Could you check a few things on this model? Use its own coordinates, in mm. Face numbers are marked on the shaded views. A direction names the side the tool comes from. Round coordinates to 2 decimals unless told otherwise and drop trailing zeros. Write each loop counter-clockwise with the first axis right and the second up, starting at its lowest first coordinate (ties: lowest second). Pieces come first, ordered by that corner, then holes. Notation, with made-up numbers: (42, 2) -> (89, 2) arc R21 ccw to (89, 30) -> close; hole circle Ø9 at (-3.75, -3.75). An arc over 180 degrees is marked (long way). Answer as CSV lines item,"result". Start each with the question number.
Q1. Imagine slicing it at B-B on y = -26.2. Please give me the cut outline in (x, z).
Q2. If we mould it in two halves opening along Y, with no side actions, what happens to the marked faces 1, 2 and 3? For each: pulls with the +Y half, pulls with the -Y half, needs draft (parallel to the pull), parting line crosses it, or undercut.
Q3. Imagine slicing it at A-A on x = 25.3. Please give me the cut outline in (y, z), and give its area (3 significant figures).
Q4. Will these pins go through, and if not, where does the flat tip stop? pin 1 Ø10.5 at (x, y) = (37, 30) entering from -Z; pin 2 Ø9 at (x, y) = (25.3, -26.2) entering from +Z; pin 3 Ø3 at (x, z) = (16.5, 1) entering from +Y; pin 4 Ø12 at (y, z) = (-4, -1) entering from +X.
Q5. Imagine slicing it at C-C on z = 0. Please give me the cut outline in (x, y).
Q6. If I drill on line 1 (X direction, y = -26, z = -6); line 2 (Y direction, x = 25.3, z = -6.6); line 3 (Z direction, x = 10.5, y = 35.5), over which ranges is the centre line in solid material (lowest first)? Write a range as [from, to].
Q7. Imagine slicing it at D-D on y = 0. Please give me the cut outline in (x, z).
Q8. For the marked faces 4, 5 and 6, which set-ups out of +Z, -Z, +X, -X, +Y, -Y let a thin tool reach every point of the face, with its end or its side?
from build123d import *

# Parameters (mm, degrees)
F0_R     = 50
F1_DEPTH = 5
F3_DEPTH = 50
F4_R     = 5
F5_DEPTH = 4


with BuildPart() as f1:
    # F0 (on Right) → F1 (new body)
    with BuildSketch(Plane.YZ):
        Circle(F0_R)
    extrude(amount=-F1_DEPTH)

    # F2 (on Right) → F3 (join)
    with BuildSketch(Plane.YZ):
        Polygon((-41.5, 9), (-41.5, -9), (41.5, -9), (41.5, 9), (16.5, 9), (16.5, 5), (37.5, 5), (37.5, -5), (-37.5, -5), (-37.5, 5), (-16.5, 5), (-16.5, 9), align=None)
    extrude(amount=F3_DEPTH)

    # F4 (on face) → F5 (cut, through all)
    with BuildSketch(Plane(origin=(0, 0, -9), x_dir=(1, 0, 0), z_dir=(0, 0, -1))):
        with Locations((25.3, 26.2)):
            Circle(F4_R)
    extrude(amount=-F5_DEPTH, mode=Mode.SUBTRACT)


solid = f1.part
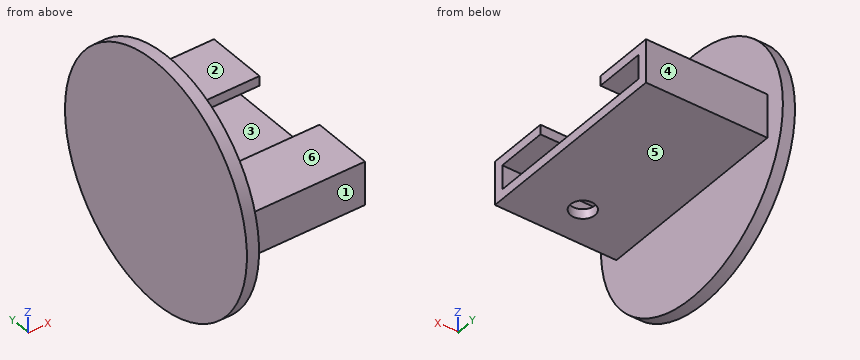
Checks:
1,outline,"(-5, -42.59) -> (0, -42.59) -> (0, -9) -> (20.3, -9) -> (20.3, -5) -> (0, -5) -> (0, 5) -> (50, 5) -> (50, 9) -> (0, 9) -> (0, 42.59) -> (-5, 42.59) -> close; (30.3, -9) -> (50, -9) -> (50, -5) -> (30.3, -5) -> close"
2,face 1,"pulls with the -Y half"
2,face 2,"needs draft"
2,face 3,"undercut"
3,outline,"(-41.5, -9) -> (-31.2, -9) -> (-31.2, -5) -> (-37.5, -5) -> (-37.5, 5) -> (-16.5, 5) -> (-16.5, 9) -> (-41.5, 9) -> close; (-21.2, -9) -> (41.5, -9) -> (41.5, 9) -> (16.5, 9) -> (16.5, 5) -> (37.5, 5) -> (37.5, -5) -> (-21.2, -5) -> close"
3,area,"572 mm^2"
4,pin 1,"z = -9"
4,pin 2,"z = 9"
4,pin 3,"y = 41.5"
4,pin 4,"x = 50"
5,outline,"(-5, -50) -> (0, -50) -> (0, -41.5) -> (50, -41.5) -> (50, -37.5) -> (0, -37.5) -> (0, 37.5) -> (50, 37.5) -> (50, 41.5) -> (0, 41.5) -> (0, 50) -> (-5, 50) -> close"
6,line 1,"[-5, 20.3], [30.3, 50]"
6,line 2,"[-41.5, -31.2], [-21.2, 41.5]"
6,line 3,"[-9, -5], [5, 9]"
7,outline,"(-5, -50) -> (0, -50) -> (0, -9) -> (50, -9) -> (50, -5) -> (0, -5) -> (0, 50) -> (-5, 50) -> close"
8,face 4,"+Z, -Z, +X, +Y"
8,face 5,"-Z, +X, +Y, -Y"
8,face 6,"+Z, +X, +Y, -Y"
